Design review of the part built by this model. Coordinates are the model's own, in mm. A direction names the side the tool comes from. Give positions to 0.01 mm unless a question says otherwise; leave off trailing zeros. Write each loop counter-clockwise with the first axis right and the second up, starting at its lowest first coordinate (ties: lowest second). Pieces come first, ordered by that corner, then holes. Notation, with made-up numbers: (-28, 42) -> (8, 42) arc R16 cw to (8, 53) -> close; hole circle Ø5 at (77, -3.5). An arc over 180 degrees is marked (long way). Write each question's results on one line, items separated by ' | '. Start each with the question number.
(1) To check wall thickness, follow probe 1 along Z at (x, y) = (2979.5, 939); probe 2 along Y at (x, z) = (2916.5, 4.5); probe 3 along X at (y, z) = (910, 8.5). State the ranges of each line that lie inside material, in increasing order.
(2) Take a section at B-B (x = 2987). State the section outline as (y, z) points.
(3) Take a section at A-A (z = 7.25). State the section outline as (x, y) points, plus the area to 3 significant figures.
(4) Mouldability with a two-part tool opening along X and no side actions: class faces 1 (the face through (2961.24, 972.59, 7.52)), 2 (the face through (2941.77, 915.47, 7.52)), 3 (the face through (2975.295, 973.772, 5.451)) as released by +X, released by -X, zero draft, split by the parting line, or undercut.
(5) Take a section at D-D (x = 2932). State the section outline as (y, z) points, plus the area to 3 significant figures.
(6) Take a section at C-C (y = 925.5). State the section outline as (x, z) points.
(7) Clearance check with flat-ended pins moving along their axes: pin 1 (2 mm diameter, centred on y = 923.5, z = 6.5, fed in from +X); pin 2 (1.5 mm diameter, centred on x = 2912.5, y = 909, fed in from +Z); pin 3 (2.5 mm diameter, centred on x = 2981.5, z = 7.5, fed in from -Y); pin 4 (2.5 mm diameter, centred on x = 2985, z = 8, fed in from +Y). State where each tip first meets the part, or that it passes through.
(8) For faces 4 (the face through (2981, 932, 6)), 5 (the face through (2941.046, 946.73, 7.521)), 6 (the face through (2961.07, 889.73, 7.52)), 7 (the face through (2974.788, 972.894, 0.986)), list the 3-axis set-ups (+Z, -Z, +X, -X, +Y, -Y) from which the entire face can be reached by the end or side of a thin tool; tool diameter is ignored.
from build123d import *

# Parameters (mm, degrees)
SKETCH1_R           = 2.6
SKETCH1_R_2         = 2.5
BOSS_EXTRUDE2_DEPTH = 9
CHAMFER1_SIZE       = 2
SKETCH3_R           = 2.6
SKETCH3_R_2         = 2.5
SKETCH3_W           = 24.934090133
SKETCH3_H           = 60
CUT_EXTRUDE1_DEPTH  = 3


with BuildPart() as part:
    # Sketch1 → Boss-Extrude2 (new body)
    with BuildSketch(Plane.XY):
        with BuildLine():
            ThreePointArc((2912.593825938, 925.76581843), (2909.393825938, 931.308381015), (2912.593825938, 936.850943599))
            Line((2912.593825938, 936.850943599), (2902.962034909, 953.533695028))
            Line((2902.962034909, 953.533695028), (2901.229984102, 952.533695028))
            Line((2901.229984102, 952.533695028), (2901.229984102, 910.083067001))
            Line((2901.229984102, 910.083067001), (2902.962034909, 909.083067001))
            Line((2902.962034909, 909.083067001), (2912.593825938, 925.76581843))
        make_face()
        with BuildLine():
            Line((2902.962034909, 953.533695028), (2912.593825938, 936.850943599))
            ThreePointArc((2912.593825938, 936.850943599), (2909.393825938, 931.308381015), (2912.593825938, 925.76581843))
            Line((2912.593825938, 925.76581843), (2902.962034909, 909.083067001))
            Line((2902.962034909, 909.083067001), (2954.923559136, 879.083067001))
            Line((2954.923559136, 879.083067001), (2964.555350165, 895.76581843))
            ThreePointArc((2964.555350165, 895.76581843), (2970.955350165, 895.76581843), (2974.155350165, 901.308381015))
            Line((2974.155350165, 901.308381015), (2993.418932222, 901.308381015))
            Line((2993.418932222, 901.308381015), (2993.418932222, 961.308381015))
            Line((2993.418932222, 961.308381015), (2974.155350165, 961.308381015))
            ThreePointArc((2974.155350165, 961.308381015), (2970.955350165, 966.850943599), (2964.555350165, 966.850943599))
            Line((2964.555350165, 966.850943599), (2954.923559136, 983.533695028))
            Line((2954.923559136, 983.533695028), (2902.962034909, 953.533695028))
        make_face()
        with Locations((2915.372288947, 910.57825753)):
            Circle(SKETCH1_R, mode=Mode.SUBTRACT)
        with Locations((2937.692797023, 909.238511568)):
            Circle(SKETCH1_R_2, mode=Mode.SUBTRACT)
        with Locations((2950.013305099, 890.57825753)):
            Circle(SKETCH1_R_2, mode=Mode.SUBTRACT)
        with Locations((2985.918932222, 911.308381015)):
            Circle(SKETCH1_R_2, mode=Mode.SUBTRACT)
        with Locations((2915.372288947, 952.0385045)):
            Circle(SKETCH1_R, mode=Mode.SUBTRACT)
        with BuildLine():
            Line((2920.935519946, 935.119284152), (2961.884164232, 958.760994954))
            ThreePointArc((2961.884164232, 958.760994954), (2964.555350165, 955.76581843), (2968.484842089, 954.950091816))
            Line((2968.484842089, 954.950091816), (2968.484842089, 907.666670213))
            ThreePointArc((2968.484842089, 907.666670213), (2964.555350165, 906.850943599), (2961.884164232, 903.855767076))
            Line((2961.884164232, 903.855767076), (2920.935519946, 927.497477877))
            ThreePointArc((2920.935519946, 927.497477877), (2922.193825938, 931.308381015), (2920.935519946, 935.119284152))
        make_face(mode=Mode.SUBTRACT)
        with Locations((2937.692797023, 953.378250462)):
            Circle(SKETCH1_R_2, mode=Mode.SUBTRACT)
        with Locations((2975.918932222, 931.308381015)):
            Circle(SKETCH1_R_2, mode=Mode.SUBTRACT)
        with Locations((2985.918932222, 951.308381015)):
            Circle(SKETCH1_R_2, mode=Mode.SUBTRACT)
        with Locations((2950.013305099, 972.0385045)):
            Circle(SKETCH1_R_2, mode=Mode.SUBTRACT)
        with BuildLine():
            Line((2956.655609944, 984.533695028), (2954.923559136, 983.533695028))
            Line((2954.923559136, 983.533695028), (2964.555350165, 966.850943599))
            ThreePointArc((2964.555350165, 966.850943599), (2970.955350165, 966.850943599), (2974.155350165, 961.308381015))
            Line((2974.155350165, 961.308381015), (2993.418932222, 961.308381015))
            Line((2993.418932222, 961.308381015), (2993.418932222, 963.308381015))
            Line((2993.418932222, 963.308381015), (2956.655609944, 984.533695028))
        make_face()
        with BuildLine():
            ThreePointArc((2961.884164232, 958.760994954), (2964.555350165, 955.76581843), (2968.484842089, 954.950091816))
            Line((2968.484842089, 954.950091816), (2968.484842089, 907.666670213))
            ThreePointArc((2968.484842089, 907.666670213), (2964.555350165, 906.850943599), (2961.884164232, 903.855767076))
            Line((2961.884164232, 903.855767076), (2920.935519946, 927.497477877))
            ThreePointArc((2920.935519946, 927.497477877), (2922.193825938, 931.308381015), (2920.935519946, 935.119284152))
            Line((2920.935519946, 935.119284152), (2961.884164232, 958.760994954))
        make_face()
        with BuildLine():
            Line((2964.555350165, 895.76581843), (2954.923559136, 879.083067001))
            Line((2954.923559136, 879.083067001), (2956.655609944, 878.083067001))
            Line((2956.655609944, 878.083067001), (2993.418932222, 899.308381015))
            Line((2993.418932222, 899.308381015), (2993.418932222, 901.308381015))
            Line((2993.418932222, 901.308381015), (2974.155350165, 901.308381015))
            ThreePointArc((2974.155350165, 901.308381015), (2970.955350165, 895.76581843), (2964.555350165, 895.76581843))
        make_face()
    extrude(amount=BOSS_EXTRUDE2_DEPTH)

    # Chamfer1
    chamfer1_edges = [part.edges().sort_by_distance(p)[0] for p in [
        (2975.037271083, 888.695724008, 0),
        (2928.942797023, 894.083067001, 0),
        (2901.229984102, 931.308381015, 0),
        (2928.942797023, 968.533695028, 0),
        (2975.037271083, 973.921038021, 0),
        (2993.418932222, 931.308381015, 0),
    ]]
    chamfer(chamfer1_edges, length=CHAMFER1_SIZE)

    # Sketch3 → Cut-Extrude1 (cut)
    with BuildSketch(Plane.XY.offset(9)):
        Polygon((2902.962034909, 909.083067001), (2954.923559136, 879.083067001), (2967.390604203, 900.676622476), (2915.429079976, 930.676622476), align=None)
        with Locations((2915.372288947, 910.57825753)):
            Circle(SKETCH3_R, mode=Mode.SUBTRACT)
        with Locations((2937.692797023, 909.238511568)):
            Circle(SKETCH3_R_2, mode=Mode.SUBTRACT)
        with Locations((2950.013305099, 890.57825753)):
            Circle(SKETCH3_R_2, mode=Mode.SUBTRACT)
        Polygon((2967.390604203, 961.940139553), (2954.923559136, 983.533695028), (2902.962034909, 953.533695028), (2915.429079976, 931.940139553), align=None)
        with Locations((2915.372288947, 952.0385045)):
            Circle(SKETCH3_R, mode=Mode.SUBTRACT)
        with Locations((2937.692797023, 953.378250462)):
            Circle(SKETCH3_R_2, mode=Mode.SUBTRACT)
        with Locations((2950.013305099, 972.0385045)):
            Circle(SKETCH3_R_2, mode=Mode.SUBTRACT)
        with Locations((2980.951887156, 931.308381015)):
            Rectangle(SKETCH3_W, SKETCH3_H)
        with Locations((2985.918932222, 911.308381015)):
            Circle(SKETCH3_R_2, mode=Mode.SUBTRACT)
        with Locations((2975.918932222, 931.308381015)):
            Circle(SKETCH3_R_2, mode=Mode.SUBTRACT)
        with Locations((2985.918932222, 951.308381015)):
            Circle(SKETCH3_R_2, mode=Mode.SUBTRACT)
    extrude(amount=-CUT_EXTRUDE1_DEPTH, mode=Mode.SUBTRACT)


solid = part.part
Report:
1) probe 1: 0 to 6 | probe 2: 901.27 to 908.24, 912.92 to 949.7, 954.38 to 961.35 | probe 3: 2901.37 to 2903.49, 2951.24 to 2968.48
2) outline: (895.6, 2) -> (897.91, 0) -> (909.05, 0) -> (909.05, 6) -> (901.31, 6) -> (901.31, 9) -> (895.6, 9) -> close; (913.56, 0) -> (949.05, 0) -> (949.05, 6) -> (913.56, 6) -> close; (953.56, 0) -> (964.7, 0) -> (967.01, 2) -> (967.01, 9) -> (961.31, 9) -> (961.31, 6) -> (953.56, 6) -> close
3) outline: (2901.23, 910.08) -> (2902.96, 909.08) -> (2915.43, 930.68) -> (2967.39, 900.68) -> (2954.92, 879.08) -> (2956.66, 878.08) -> (2993.42, 899.31) -> (2993.42, 901.31) -> (2968.48, 901.31) -> (2968.48, 961.31) -> (2993.42, 961.31) -> (2993.42, 963.31) -> (2956.66, 984.53) -> (2954.92, 983.53) -> (2967.39, 961.94) -> (2915.43, 931.94) -> (2902.96, 953.53) -> (2901.23, 952.53) -> close | area: 2,770 mm2
4) face 1: released by -X | face 2: undercut | face 3: released by +X
5) outline: (892.32, 2) -> (894.63, 0) -> (967.99, 0) -> (970.3, 2) -> (970.3, 6) -> (941.51, 6) -> (941.51, 9) -> (921.11, 9) -> (921.11, 6) -> (892.32, 6) -> close | area: 524 mm2
6) outline: (2901.23, 2) -> (2903.23, 0) -> (2991.42, 0) -> (2993.42, 2) -> (2993.42, 6) -> (2968.48, 6) -> (2968.48, 9) -> (2924.4, 9) -> (2924.4, 6) -> (2912.44, 6) -> (2912.44, 9) -> (2901.23, 9) -> close
7) pin 1: x = 2993.42 | pin 2: z = 6 | pin 3: y = 891.71 | pin 4: y = 968.89
8) face 4: +Z, +X | face 5: +Z | face 6: +Z, -X | face 7: -Z, +X, +Y
